Input: part model. Units: mm. Frame: model coordinates. Face numbers are marked on the shaded views. A direction names the side the tool comes from. Round coordinates to 2 decimals unless told otherwise and drop trailing zeros. Order: outer loops, then holes, each group sorted by start corner. A loop starts at its lowest first (then second) coordinate and runs counter-clockwise, first axis right, second up. Notation, with made-up numbers: (66.25, 17.25) -> (93.25, 17.25) arc R16 ccw to (93.25, 24.25) -> close; hole circle Ø5 at (86.5, 22). An arc over 180 degrees is marked (long way). Use a Markdown table: item, result.
from build123d import *

# Parameters (mm, degrees)
EXTRUDE_1_DEPTH     = 111
SKETCH_3_W          = 12
SKETCH_3_H          = 25
CUT_EXTRUDE_1_DEPTH = 2
SKETCH_5_W          = 12
SKETCH_5_H          = 25
CUT_EXTRUDE_2_DEPTH = 2
SKETCH_6_W          = 5
SKETCH_6_H          = 99
CUT_EXTRUDE_3_DEPTH = 2


with BuildPart() as part:
    # 草圖1 → 填料-伸長1 (new body)
    with BuildSketch(Plane(origin=(0, 0, 0), x_dir=(1, 0, 0), z_dir=(0, 1, 0))):
        Polygon((-15, 5.665584657), (65, 5.665584657), (80, -20.315177457), (65, -20.315177457), (-15, -20.315177457), (-30, -20.315177457), align=None)
        Polygon((-13.845299462, 3.665584657), (63.845299462, 3.665584657), (76.535898385, -18.315177457), (65, -18.315177457), (-15, -18.315177457), (-26.535898385, -18.315177457), align=None, mode=Mode.SUBTRACT)
    extrude(amount=EXTRUDE_1_DEPTH)

    # 草圖3 → 除料-伸長1 (cut)
    with BuildSketch(Plane(origin=(51.20327012, 0, -29.562221787), x_dir=(-0.5, 0, -0.866025404), z_dir=(0.866025404, 0, -0.5))):
        with Locations((-37.59345976, 92.5)):
            Rectangle(SKETCH_3_W, SKETCH_3_H)
        with Locations((-37.59345976, 55.5)):
            Rectangle(SKETCH_3_W, SKETCH_3_H)
        with Locations((-37.59345976, 18.5)):
            Rectangle(SKETCH_3_W, SKETCH_3_H)
    extrude(amount=-CUT_EXTRUDE_1_DEPTH, mode=Mode.SUBTRACT)

    # 草圖5 → 除料-伸長2 (cut)
    with BuildSketch(Plane(origin=(-13.70327012, 0, -7.911586693), x_dir=(-0.5, 0, 0.866025404), z_dir=(-0.866025404, 0, -0.5))):
        with Locations((12.59345976, 92.5)):
            Rectangle(SKETCH_5_W, SKETCH_5_H)
        with Locations((12.59345976, 55.5)):
            Rectangle(SKETCH_5_W, SKETCH_5_H)
        with Locations((12.59345976, 18.5)):
            Rectangle(SKETCH_5_W, SKETCH_5_H)
    extrude(amount=-CUT_EXTRUDE_2_DEPTH, mode=Mode.SUBTRACT)

    # 草圖6 → 除料-伸長3 (cut)
    with BuildSketch(Plane(origin=(0, 0, -5.665584657), x_dir=(-1, 0, 0), z_dir=(0, 0, -1))):
        with Locations((-58.5, 55.5)):
            Rectangle(SKETCH_6_W, SKETCH_6_H)
        with Locations((8.5, 55.5)):
            Rectangle(SKETCH_6_W, SKETCH_6_H)
    extrude(amount=-CUT_EXTRUDE_3_DEPTH, mode=Mode.SUBTRACT)


solid = part.part
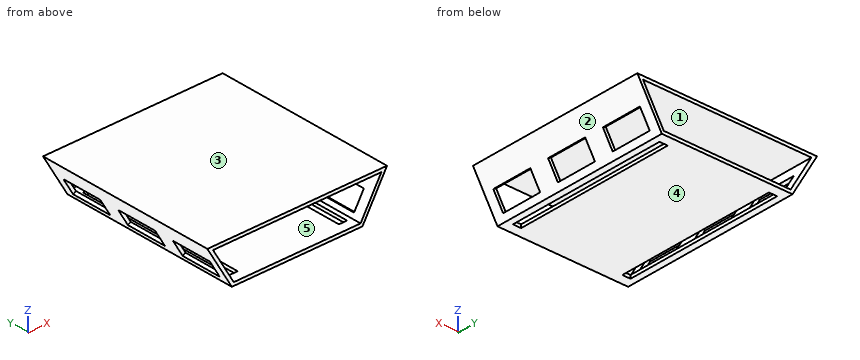
1) Ray query, probe 1 along Z at (x, y) = (49.5, 29.5); probe 2 along X at (y, z) = (64.5, 10.25); probe 3 along X at (y, z) = (60, 13). Return the intervals inside material, ascending.
Answer key:
| item | result |
|---|---|
| probe 1 | z = -5.67 to -3.67, 18.32 to 20.32 |
| probe 2 | x = -24.19 to -21.88, 71.88 to 74.19 |
| probe 3 | x = -25.78 to -23.47, 73.47 to 75.78 |
2) Cut plane B-B on y = 84. Return loops of the section in (x, z), and give its area (3 significant figures).
Answer key:
| item | result |
|---|---|
| outline | (-30, 20.32) -> (-23, 8.19) -> (-21.27, 9.19) -> (-26.54, 18.32) -> (76.54, 18.32) -> (71.27, 9.19) -> (73, 8.19) -> (80, 20.32) -> close; (-17, -2.2) -> (-15, -5.67) -> (-11, -5.67) -> (-11, -3.67) -> (-13.85, -3.67) -> (-15.27, -1.2) -> close; (-6, -5.67) -> (56, -5.67) -> (56, -3.67) -> (-6, -3.67) -> close; (61, -5.67) -> (65, -5.67) -> (67, -2.2) -> (65.27, -1.2) -> (63.85, -3.67) -> (61, -3.67) -> close |
| area | 414 mm^2 |
3) Cut plane A-A on x = 27. Return loops of the section in (y, z).
Answer key:
| item | result |
|---|---|
| outline | (0, -5.67) -> (111, -5.67) -> (111, -3.67) -> (0, -3.67) -> close; (0, 18.32) -> (111, 18.32) -> (111, 20.32) -> (0, 20.32) -> close |
4) Set-up query: the marked faces 4 and 5. Return all of +Z, -Z, +X, -X, +Y, -Y with unobstructed straight access to the full face (end or side cutting, diameter ignored); none if empty.
Answer key:
| item | result |
|---|---|
| face 4 | -Z, +X, -X, +Y, -Y |
| face 5 | +Y, -Y |
5) Cut plane C-C on z = 2. State how many separate pieces and enclosed holes the cut face has, and give its area (3 significant figures).
Answer key:
| item | result |
|---|---|
| separate pieces | 8 |
| enclosed holes | 0 |
| area | 166 mm^2 |
6) Contact query for flat-ended pins moving along their axis: P1, Ø10, axis at x = -8, z = 9.5, coming from the -Y side; P2, Ø3, axis at y = 82.5, z = 7, coming from the +X side; P3, Ø10, axis at y = 46.5, z = 8, coming from the -X side; P4, Ø2, axis at y = 65, z = -4.5, coming from the -X side. Output: stop coordinate, or through.
Answer key:
| item | result |
|---|---|
| P1 | passes through |
| P2 | stops at x = 73.18 |
| P3 | stops at x = -25.78 |
| P4 | stops at x = -16.25 |
7) Cut plane D-D on y = 40. Return loops of the section in (x, z), and give its area (3 significant figures).
Answer key:
| item | result |
|---|---|
| outline | (-30, 20.32) -> (-15, -5.67) -> (-11, -5.67) -> (-11, -3.67) -> (-13.85, -3.67) -> (-26.54, 18.32) -> (76.54, 18.32) -> (63.85, -3.67) -> (61, -3.67) -> (61, -5.67) -> (65, -5.67) -> (80, 20.32) -> close; (-6, -5.67) -> (56, -5.67) -> (56, -3.67) -> (-6, -3.67) -> close |
| area | 462 mm^2 |
8) Draft query along Z for the marked faces 1, 2 and 3. Return one class per face: released by +Z, released by -Z, zero draft, split by the parting line, or undercut.
Answer key:
| item | result |
|---|---|
| face 1 | undercut |
| face 2 | released by -Z |
| face 3 | released by +Z |
